Geometry check sheet. Reference: the model listing, model coordinates, mm. Give positions to 0.01 mm unless a question says otherwise; leave off trailing zeros. Loops run counter-clockwise (first coordinate to the right, second up) from the corner with the lowest first, then second, coordinate; pieces in that order, holes last.
1. Cross-section at A-A, the plane z = 35. Record the cut outline in (x, y) (3 decimals).
2. Go/stop test with flat-tipped pins: pin 1 Ø0.6 at (y, z) = (8.5, 78.5) entering from +X; pin 2 Ø4 at (y, z) = (-5, 112) entering from +X; pin 3 Ø1.5 at (y, z) = (-6, 85.5) entering from +X; pin 4 Ø5 at (x, y) = (-1.5, -1) entering from -Z. Record where each tip stops, or that it passes through.
3. Material ranges on L1, parallel to Y at x = -0.5, z = 46.5; L2, parallel to Y at x = -5, z = 27.5; L3, parallel to X at y = 4.25, z = 69, recorded low to high.
4. Cross-section at B-B, the plane x = -4.5. Record the cut outline in (y, z).
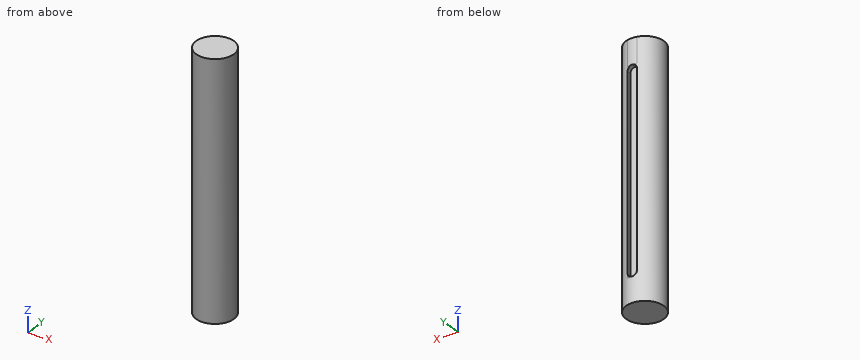
from build123d import *
from build123d.topology import SkipClean

# Parameters (mm, degrees)
SKETCH1_R          = 9.525
EXTRUDE1_DEPTH     = 127
SKETCH2_W          = 4.7625
SKETCH2_H          = 4.7625
CUT_EXTRUDE1_DEPTH = 114.3
EXTRUDE2_START     = -12.7
EXTRUDE2_DEPTH     = 12.7
FILLET1_R          = 2.38125


with BuildPart() as part:
    # Sketch1 → Extrude1 (new body)
    with BuildSketch(Plane.XY):
        Circle(SKETCH1_R)
    extrude(amount=EXTRUDE1_DEPTH)

    # Sketch2 → Cut-Extrude1 (cut)
    with BuildSketch(Plane.XY.offset(127)):
        with Locations((0, 9.525)):
            Rectangle(SKETCH2_W, SKETCH2_H)
    extrude(amount=-CUT_EXTRUDE1_DEPTH, mode=Mode.SUBTRACT)

    # Sketch4 → Extrude2 (add)
    with SkipClean():  # the faces are left unmerged after this step: merging them gives an invalid solid
        with BuildSketch(Plane.XY.offset(127).offset(EXTRUDE2_START)):
            with BuildLine():
                Line((2.38125, 7.14375), (-2.38125, 7.14375))
                Line((-2.38125, 7.14375), (-2.38125, 9.222541593))
                ThreePointArc((-2.38125, 9.222541593), (0, 9.525), (2.38125, 9.222541593))
                Line((2.38125, 9.222541593), (2.38125, 7.14375))
            make_face()
        extrude(amount=EXTRUDE2_DEPTH)

    # Fillet1
    # the kernel refuses this fillet: 2.38125 mm, written as the material it adds along each edge
    with BuildSketch(Plane(origin=(2.38125, 15.175666593, 114.3), x_dir=(0, 0, -1), z_dir=(0, -1, 0))) as fillet1_piece_1_section:
        with BuildLine():
            CenterArc((FILLET1_R, -FILLET1_R), FILLET1_R, 90, 90)
            Line((0, -FILLET1_R), (0, 0))
            Line((0, 0), (FILLET1_R, 0))
        make_face()
    fillet1_piece_1 = extrude(amount=13.985041593, mode=Mode.PRIVATE)
    fillet1_piece_1 = fillet1_piece_1 & Plane(origin=(0, 0, 113.773698621), x_dir=(1, 0, 0), z_dir=(0, 0, -1)) * Cylinder(9.525, 38, mode=Mode.PRIVATE)
    add(fillet1_piece_1)
    with BuildSketch(Plane(origin=(-2.38125, 1.190625, 114.3), x_dir=(0, 0, -1), z_dir=(0, 1, 0))) as fillet1_piece_2_section:
        with BuildLine():
            CenterArc((FILLET1_R, -FILLET1_R), FILLET1_R, 90, 90)
            Line((0, -FILLET1_R), (0, 0))
            Line((0, 0), (FILLET1_R, 0))
        make_face()
    fillet1_piece_2 = extrude(amount=13.985041593, mode=Mode.PRIVATE)
    fillet1_piece_2 = fillet1_piece_2 & Plane(origin=(0, 0, 113.760896634), x_dir=(1, 0, 0), z_dir=(0, 0, -1)) * Cylinder(9.525, 38, mode=Mode.PRIVATE)
    add(fillet1_piece_2)
    with BuildSketch(Plane(origin=(-2.38125, 1.190625, 12.7), x_dir=(0, 0, 1), z_dir=(0, 1, 0))) as fillet1_piece_3_section:
        with BuildLine():
            CenterArc((FILLET1_R, FILLET1_R), FILLET1_R, 180, 90)
            Line((0, FILLET1_R), (0, 0))
            Line((0, 0), (FILLET1_R, 0))
        make_face()
    fillet1_piece_3 = extrude(amount=13.985041593, mode=Mode.PRIVATE)
    fillet1_piece_3 = fillet1_piece_3 & Plane(origin=(0, 0, 13.239103366), x_dir=(1, 0, 0), z_dir=(0, 0, -1)) * Cylinder(9.525, 38, mode=Mode.PRIVATE)
    add(fillet1_piece_3)
    with BuildSketch(Plane(origin=(2.38125, 15.175666593, 12.7), x_dir=(-1, 0, 0), z_dir=(0, -1, 0))) as fillet1_piece_4_section:
        with BuildLine():
            CenterArc((FILLET1_R, -FILLET1_R), FILLET1_R, 90, 90)
            Line((0, -FILLET1_R), (0, 0))
            Line((0, 0), (FILLET1_R, 0))
        make_face()
    fillet1_piece_4 = extrude(amount=13.985041593, mode=Mode.PRIVATE)
    fillet1_piece_4 = fillet1_piece_4 & Plane(origin=(0, 0, 13.226300129), x_dir=(1, 0, 0), z_dir=(0, 0, -1)) * Cylinder(9.525, 38, mode=Mode.PRIVATE)
    add(fillet1_piece_4)


solid = part.part
Result:
1. outline: (-2.381, 7.144) - (-2.381, 9.223) arc R9.525 ccw (long way) to (2.381, 9.223) - (2.381, 7.144) - close
2. pin 1: stops at x = 4.85
2. pin 2: stops at x = 9.04
2. pin 3: stops at x = 7.95
2. pin 4: stops at z = 0
3. L1: y = -9.51 to 7.14
3. L2: y = -8.11 to 8.11
3. L3: x = -8.52 to 8.52
4. outline: (-8.39, 0) - (8.39, 0) - (8.39, 127) - (-8.39, 127) - close
